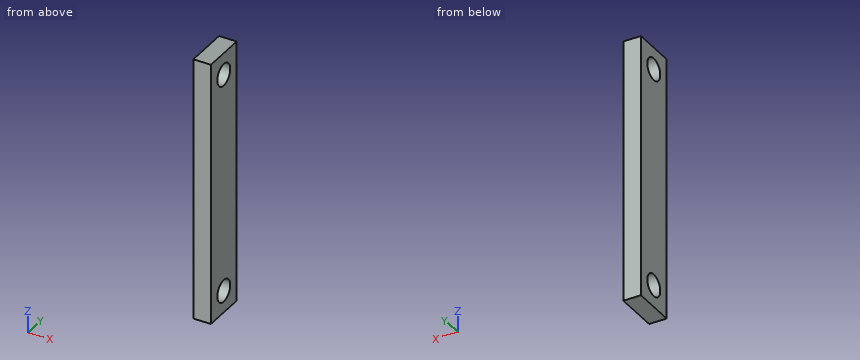
Autodesk Inventor part; units mm, degrees
ref_plane "作業平面1" through (0, 2.5, -15) normal (-1, 0, 0) x (0, 0, 1)
ref_plane "YZ Plane" through (0, 0, 0) normal (1, 0, 0) x (0, 1, 0)
ref_plane "XZ Plane" through (0, 0, 0) normal (0, 1, 0) x (-1, 0, 0)
sketch "スケッチ1" plane through (0, 0, 0) normal (0, 1, 0) x (-1, 0, 0)
  line L0 (2, -15) -> (2, 15)
  line L1 (-2, -15) -> (2, 15) construction
  line L2 (2, -15) -> (-2, 15) construction
  line L3 (0, -15) -> (0, 15)
  line L4 (0, -15) -> (2, -15)
  line L5 (2, 15) -> (0, 15)
  point P0 (0, 0)
  dimension "d1" = 30
  dimension "d33" = 2
extrude "押し出し1" add sketch "スケッチ1" along normal mid plane 5
sketch "スケッチ2" plane through (0, 2.5, 0) normal (0, 1, 0) x (1, 0, 0)
  line L0 (-2, -15) -> (2, -15)
  line L1 (0, -15) -> (2, -15)
  line L2 (2, -15) -> (2, -5)
  line L3 (2, -5) -> (0, -5)
  line L4 (0, -5) -> (0, -15)
  point P0 (0, 0)
  dimension "d4" = 2
  dimension "d5" = 10
extrude "押し出し2" cut sketch "スケッチ2" against normal blind 5
sketch "スケッチ4" plane through (0, 2.5, 15) normal (1, 0, 0) x (0, 0, -1)
  circle A0 centre (2.5, -2.5) radius 1.25
  point P0 (15, -2.5)
  dimension "d12" = 2.5
extrude "押し出し4" cut sketch "スケッチ4" against normal blind 5
ref_plane "作業平面1" through (0, 2.5, -15) normal (-1, 0, 0) x (0, 0, 1)
sketch "スケッチ5" plane through (0, 2.5, -15) normal (-1, 0, 0) x (0, 0, 1)
  circle A0 centre (2.5, -2.5) radius 1.25
  point P0 (15, -2.5)
  dimension "d15" = 2.5
extrude "押し出し5" cut sketch "スケッチ5" along normal mid plane 5
properties part number "promo_arm2"
Work out the finished part from the listing and answer in its coordinate system (mm). Give positions to 0.01 mm unless a question says otherwise; leave off trailing zeros. Write each loop counter-clockwise with the first axis right and the second up, starting at its lowest first coordinate (ties: lowest second). Pieces come first, ordered by that corner, then holes.
Q1. Straight lines are drawn through the part: L1, parallel to Z at x = -1.1, y = 0.1; L2, parallel to Y at x = -0.75, z = -12.5; L3, parallel to Z at x = -0.8, y = -0.75. For each, find the intervals that lie inside material, in ascending order.
Answer:
L1: z = -15 to -13.75, -11.25 to 11.25, 13.75 to 15
L2: y = -2.5 to -1.25, 1.25 to 2.5
L3: z = -15 to -13.5, -11.5 to 11.5, 13.5 to 15
Q2. Given pin 1 (3 mm diameter, centred on y = 0, z = -12.5, fed in from +X), flat-ended and moving along its own axis, determine where the tip first touches the part or whether it passes through.
Answer:
pin 1: stops at x = 0
Q3. The part is cut by section A-A on y = 0. Give the vertices of the cut face in (x, z).
Answer:
outline: (-2, -15) - (0, -15) - (0, -13.75) - (-2, -13.75) - close; (-2, -11.25) - (0, -11.25) - (0, 11.25) - (-2, 11.25) - close; (-2, 13.75) - (0, 13.75) - (0, 15) - (-2, 15) - close
Q4. The part is cut by section C-C on x = -0.9. Give the vertices of the cut face in (y, z), and give its area (3 significant figures).
Answer:
outline: (-2.5, -15) - (2.5, -15) - (2.5, 15) - (-2.5, 15) - close; hole circle Ø2.5 at (0, -12.5); hole circle Ø2.5 at (0, 12.5)
area: 140 mm2
Q5. The part is cut by section B-B on z = -12.5. Give the vertices of the cut face in (x, y), and give its area (3 significant figures).
Answer:
outline: (-2, -2.5) - (0, -2.5) - (0, -1.25) - (-2, -1.25) - close; (-2, 1.25) - (0, 1.25) - (0, 2.5) - (-2, 2.5) - close
area: 5.00 mm2
